from build123d import *

# Parameters (mm, degrees)
SKETCH_1_R          = 2.85
EXTRUDE_1_DEPTH     = 4.5
EXTRUDE_2_DEPTH     = 6
SKETCH_3_R          = 3.25
EXTRUDE_3_DEPTH     = 2.5
CHAMFER_3_SIZE      = 0.2
FILLET_2_R          = 0.3
CHAMFER_4_SIZE      = 0.2
CHAMFER_5_SIZE      = 0.3
SKETCH_5_R          = 2.7
CUT_EXTRUDE_1_DEPTH = 5


with BuildPart() as part:
    # 草图1 → 凸台-拉伸1 (new body)
    with BuildSketch(Plane(origin=(0, 0, 0), x_dir=(1, 0, 0), z_dir=(0, 1, 0))):
        Circle(SKETCH_1_R)
    extrude(amount=EXTRUDE_1_DEPTH)

    # 草图2 → 凸台-拉伸2 (add)
    with BuildSketch(Plane(origin=(0, 4.5, 0), x_dir=(1, 0, 0), z_dir=(0, 1, 0))):
        Polygon((4.618802154, 0), (2.309401077, 4), (-2.309401077, 4), (-4.618802154, 0), (-2.309401077, -4), (2.309401077, -4), align=None)
    extrude(amount=EXTRUDE_2_DEPTH)

    # 草图3 → 凸台-拉伸3 (add)
    with BuildSketch(Plane(origin=(0, 10.5, 0), x_dir=(1, 0, 0), z_dir=(0, 1, 0))):
        Circle(SKETCH_3_R)
    extrude(amount=EXTRUDE_3_DEPTH)

    # 倒角3
    chamfer_3_edges = [part.edges().sort_by_distance(p)[0] for p in [
        (-2.85, 4.5, 0),
        (3.464101615, 4.5, 2),
        (3.464101615, 4.5, -2),
        (0, 4.5, -4),
        (-3.464101615, 4.5, -2),
        (-3.464101615, 4.5, 2),
        (0, 4.5, 4),
    ]]
    chamfer(chamfer_3_edges, length=CHAMFER_3_SIZE)

    # 圆角2
    fillet_2_edges = [part.edges().sort_by_distance(p)[0] for p in [
        (-3.25, 10.5, 0),
        (3.464101615, 10.5, 2),
        (3.464101615, 10.5, -2),
        (0, 10.5, -4),
        (-3.464101615, 10.5, -2),
        (-3.464101615, 10.5, 2),
        (0, 10.5, 4),
    ]]
    fillet(fillet_2_edges, radius=FILLET_2_R)

    # 倒角4
    chamfer_4_edges = [part.edges().sort_by_distance(p)[0] for p in [
        (-3.25, 13, 0),
    ]]
    chamfer(chamfer_4_edges, length=CHAMFER_4_SIZE)

    # 倒角5
    chamfer_5_edges = [part.edges().sort_by_distance(p)[0] for p in [
        (-2.85, 0, 0),
    ]]
    chamfer(chamfer_5_edges, length=CHAMFER_5_SIZE)

    # 草图5 → 切除-拉伸1 (cut)
    with BuildSketch(Plane(origin=(0, 13, 0), x_dir=(1, 0, 0), z_dir=(0, 1, 0))):
        Circle(SKETCH_5_R)
    extrude(amount=-CUT_EXTRUDE_1_DEPTH, mode=Mode.SUBTRACT)


solid = part.part
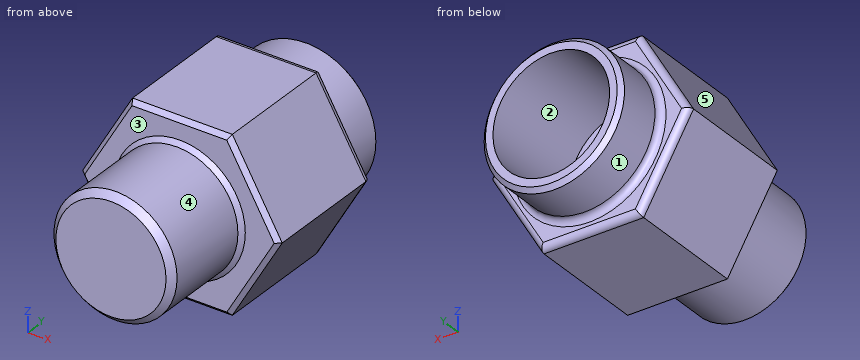
For this review, take the finished solid that the model builds, in its own axes (mm). Face numbers are marked on the shaded views. A direction names the side the tool comes from. Give positions to 0.01 mm unless a question says otherwise; leave off trailing zeros. Order: outer loops, then holes, each group sorted by start corner. A loop starts at its lowest first (then second) coordinate and runs counter-clockwise, first axis right, second up. Notation, with made-up numbers: M 69.25,79.25 L 124.25,79.25 A19 cw 124.25,109.25 Z; hole C 8.25,-27.5 d11. An arc over 180 degrees is marked long. Answer in a Markdown table with one row per item. Add a question column.
(1) Wall thickness on probe 1 along Z at (x, y) = (0, 12); probe 2 along Z at (x, y) = (0, 10.2): over which ranges is each line inside the solid? List them lowest first. Write a range as [from, to].
(2) Consider section C-C on y = 1.75. State the section outline as (x, z) points, and give its area (3 significant figures).
(3) Consider section D-D on y = 5.75. State the section outline as (x, z) points.
(4) For pin 1 (2 mm diameter, centred on y = 1.5, z = 0, fed in from +X); pin 2 (1.5 mm diameter, centred on x = 3.5, z = -2, fed in from -Y); pin 3 (2 mm diameter, centred on x = -0.5, z = 0, fed in from +Y), all flat-tipped, find the tip position at first contact; note any pin that passes through.
(5) For the marked faces 4 and 5, list the 3-axis set-ups (+Z, -Z, +X, -X, +Y, -Y) from which the entire face can be reached by the end or side of a thin tool; tool diameter is ignored.
(6) Consider section B-B on x = 0. State the section outline as (y, z) points, and give its area (3 significant figures).
(7) Mouldability with a two-part tool opening along Z and no side actions: class the marked faces 1, 2 and 3 as +Z half, -Z half, draft (parallel to the pull), parting line (faces both ways), or undercut.
(8) Consider section A-A on y = 9.75. State the section outline as (x, z) points.
Evaluation:
| question | item | result |
|---|---|---|
| 1 | probe 1 | z = [-3.25, -2.7], [2.7, 3.25] |
| 1 | probe 2 | z = [-4, -2.7], [2.7, 4] |
| 2 | outline | C 0,0 d5.7 |
| 2 | area | 25.5 mm^2 |
| 3 | outline | M -4.62,0 L -2.31,-4 L 2.31,-4 L 4.62,0 L 2.31,4 L -2.31,4 Z |
| 4 | pin 1 | stops at x = 2.85 |
| 4 | pin 2 | stops at y = 4.5 |
| 4 | pin 3 | stops at y = 8 |
| 5 | face 4 | -Y |
| 5 | face 5 | +Z, -X, +Y, -Y |
| 6 | outline | M 0,-2.55 L 0.3,-2.85 L 4.3,-2.85 L 4.5,-3.05 L 4.5,-3.8 L 4.7,-4 L 10.2,-4 A0.3 ccw 10.5,-3.7 L 10.5,-3.55 A0.3 cw 10.8,-3.25 L 12.8,-3.25 L 13,-3.05 L 13,-2.7 L 8,-2.7 L 8,2.7 L 13,2.7 L 13,3.05 L 12.8,3.25 L 10.8,3.25 A0.3 cw 10.5,3.55 L 10.5,3.7 A0.3 ccw 10.2,4 L 4.7,4 L 4.5,3.8 L 4.5,3.05 L 4.3,2.85 L 0.3,2.85 L 0,2.55 Z |
| 6 | area | 62.8 mm^2 |
| 7 | face 1 | parting line |
| 7 | face 2 | undercut |
| 7 | face 3 | draft |
| 8 | outline | M -4.62,0 L -2.31,-4 L 2.31,-4 L 4.62,0 L 2.31,4 L -2.31,4 Z; hole C 0,0 d5.4 |
